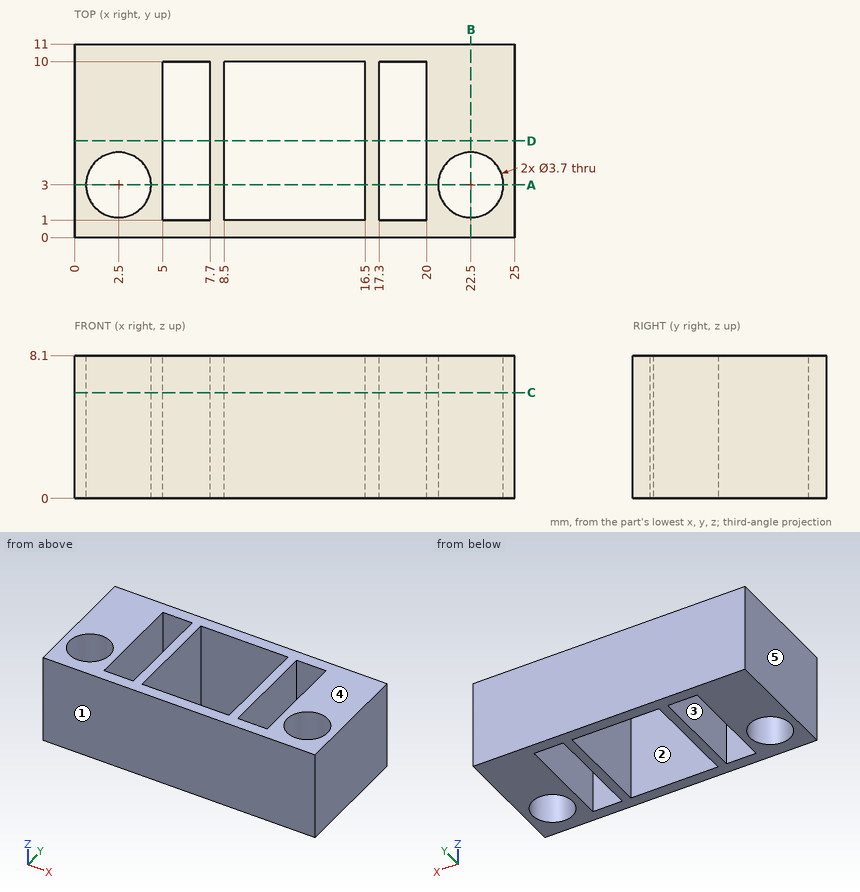
Design review of the part shown in the three views and the two pictorial views. Dimensions are in mm from the part's minimum x, y and z. A direction names the side the tool comes from. Round coordinates to 2 decimals unless told otherwise and drop trailing zeros. Write each loop counter-clockwise with the first axis right and the second up, starting at its lowest first coordinate (ties: lowest second). Pieces come first, ordered by that corner, then holes. Notation, with made-up numbers: (-33.5, -13.5) -> (-28.5, -13.5) arc R30 ccw to (-28.5, 22.5) -> close; hole circle Ø6 at (66.25, 72.25). An arc over 180 degrees is marked (long way). Use one line per item in the form item = value.
1) Take a section at D-D, the plane y = 5.5. Write out the cut boundary in (x, z), and give its area (3 significant figures).
Found:
outline = (0, 0) -> (5, 0) -> (5, 8.1) -> (0, 8.1) -> close; (7.7, 0) -> (8.5, 0) -> (8.5, 8.1) -> (7.7, 8.1) -> close; (16.5, 0) -> (17.3, 0) -> (17.3, 8.1) -> (16.5, 8.1) -> close; (20, 0) -> (25, 0) -> (25, 8.1) -> (20, 8.1) -> close
area = 94.0 mm2
2) Mouldability with a two-part tool opening along X and no side actions: class the marked faces 3, 4 and 5 as +X half, -X half, draft (parallel to the pull), parting line (faces both ways), or undercut.
Found:
face_3 = undercut
face_4 = draft
face_5 = -X half
3) Tool access review of the marked faces 1 and 2: name each direction out of +Z, -Z, +X, -X, +Y, -Y from which nothing blocks a thin tool from reaching the whole face with its end or side.
Found:
face_1 = +Z, -Z, +X, -X, -Y
face_2 = +Z, -Z
4) Take a section at B-B, the plane x = 22.5. Write out the cut boundary in (y, z), and give its area (3 significant figures).
Found:
outline = (0, 0) -> (1.15, 0) -> (1.15, 8.1) -> (0, 8.1) -> close; (4.85, 0) -> (11, 0) -> (11, 8.1) -> (4.85, 8.1) -> close
area = 59.1 mm2
5) To check wall thickness, follow L1, parallel to X at y = 6.25, z = 5.75; L2, parallel to Y at x = 2.5, z = 5.5; L3, parallel to Y at x = 16.25, z = 3.25. State the ranges of each line that lie inside material, in increasing order. Write a range as from..to.
Found:
L1 = 0..5, 7.7..8.5, 16.5..17.3, 20..25
L2 = 0..1.15, 4.85..11
L3 = 0..1, 10..11
6) Clearance check with a flat-ended pin moving along its axis: pin 1 (2 mm diameter, centred on x = 22.5, y = 3, fed in from +Z). State where the tip first meets the part, or that it passes through.
Found:
pin_1 = through
7) Take a section at A-A, the plane y = 3. Write out the cut boundary in (x, z).
Found:
outline = (0, 0) -> (0.65, 0) -> (0.65, 8.1) -> (0, 8.1) -> close; (4.35, 0) -> (5, 0) -> (5, 8.1) -> (4.35, 8.1) -> close; (7.7, 0) -> (8.5, 0) -> (8.5, 8.1) -> (7.7, 8.1) -> close; (16.5, 0) -> (17.3, 0) -> (17.3, 8.1) -> (16.5, 8.1) -> close; (20, 0) -> (20.65, 0) -> (20.65, 8.1) -> (20, 8.1) -> close; (24.35, 0) -> (25, 0) -> (25, 8.1) -> (24.35, 8.1) -> close
8) Take a section at C-C, the plane z = 6. Write out the cut boundary in (x, y), and give its area (3 significant figures).
Found:
outline = (0, 0) -> (25, 0) -> (25, 11) -> (0, 11) -> close; hole circle Ø3.7 at (2.5, 3); hole (5, 1) -> (7.7, 1) -> (7.7, 10) -> (5, 10) -> close; hole (8.5, 1) -> (16.5, 1) -> (16.5, 10) -> (8.5, 10) -> close; hole (17.3, 1) -> (20, 1) -> (20, 10) -> (17.3, 10) -> close; hole circle Ø3.7 at (22.5, 3)
area = 133 mm2
